The model under review builds one solid part; all positions refer to its coordinate system, in mm. A direction names the side the tool comes from. Round coordinates to 2 decimals unless told otherwise and drop trailing zeros. Use CSV: the item, a comma, the result in double quotes. Start each with the question number.
```python
from build123d import *

# Parameters (mm, degrees)
SKETCH3_R           = 0.95
SKETCH3_W           = 4.2
SKETCH3_H           = 8
SKETCH3_H_2         = 6
BOSS_EXTRUDE3_DEPTH = 2


with BuildPart() as part:
    # Sketch3 → Boss-Extrude3 (new body)
    with BuildSketch(Plane.XY):
        with BuildLine():
            Line((0, 94.006448831), (0, 86.061448831))
            ThreePointArc((0, 86.061448831), (0.585786438, 84.647235269), (2, 84.061448831))
            Line((2, 84.061448831), (4, 84.061448831))
            Line((4, 84.061448831), (4, 78.061448831))
            Line((4, 78.061448831), (2, 78.061448831))
            ThreePointArc((2, 78.061448831), (0.585786438, 77.475662393), (0, 76.061448831))
            Line((0, 76.061448831), (0, 60.606448831))
            ThreePointArc((0, 60.606448831), (0.585786438, 59.192235269), (2, 58.606448831))
            Line((2, 58.606448831), (4, 58.606448831))
            Line((4, 58.606448831), (4, 50.606448831))
            Line((4, 50.606448831), (2, 50.606448831))
            ThreePointArc((2, 50.606448831), (0.585786438, 50.020662393), (0, 48.606448831))
            Line((0, 48.606448831), (0, 26.346448831))
            ThreePointArc((0, 26.346448831), (0.585786438, 24.932235269), (2, 24.346448831))
            Line((2, 24.346448831), (4, 24.346448831))
            Line((4, 24.346448831), (4, 12.346448831))
            Line((4, 12.346448831), (6, 12.346448831))
            Line((6, 12.346448831), (6, 24.346448831))
            Line((6, 24.346448831), (10.2, 24.346448831))
            Line((10.2, 24.346448831), (10.2, 12.346448831))
            Line((10.2, 12.346448831), (12.2, 12.346448831))
            Line((12.2, 12.346448831), (12.2, 24.346448831))
            Line((12.2, 24.346448831), (14.2, 24.346448831))
            ThreePointArc((14.2, 24.346448831), (15.614213562, 24.932235269), (16.2, 26.346448831))
            Line((16.2, 26.346448831), (16.2, 48.606448831))
            ThreePointArc((16.2, 48.606448831), (15.614213562, 50.020662393), (14.2, 50.606448831))
            Line((14.2, 50.606448831), (12.2, 50.606448831))
            Line((12.2, 50.606448831), (12.2, 58.606448831))
            Line((12.2, 58.606448831), (14.2, 58.606448831))
            ThreePointArc((14.2, 58.606448831), (15.614213562, 59.192235269), (16.2, 60.606448831))
            Line((16.2, 60.606448831), (16.2, 76.061448831))
            ThreePointArc((16.2, 76.061448831), (15.614213562, 77.475662393), (14.2, 78.061448831))
            Line((14.2, 78.061448831), (12.2, 78.061448831))
            Line((12.2, 78.061448831), (12.2, 84.061448831))
            Line((12.2, 84.061448831), (14.2, 84.061448831))
            ThreePointArc((14.2, 84.061448831), (15.614213562, 84.647235269), (16.2, 86.061448831))
            Line((16.2, 86.061448831), (16.2, 94.006448831))
            Line((16.2, 94.006448831), (0, 94.006448831))
        make_face()
        with Locations((6, 33.846448831)):
            Circle(SKETCH3_R, mode=Mode.SUBTRACT)
        with Locations((10.2, 33.846448831)):
            Circle(SKETCH3_R, mode=Mode.SUBTRACT)
        with Locations((2.75, 86.061448831)):
            Circle(SKETCH3_R, mode=Mode.SUBTRACT)
        with Locations((10.2, 41.166448831)):
            Circle(SKETCH3_R, mode=Mode.SUBTRACT)
        with Locations((13.45, 48.106448831)):
            Circle(SKETCH3_R, mode=Mode.SUBTRACT)
        with Locations((2.75, 92.061448831)):
            Circle(SKETCH3_R, mode=Mode.SUBTRACT)
        with Locations((13.45, 86.061448831)):
            Circle(SKETCH3_R, mode=Mode.SUBTRACT)
        with Locations((2.75, 61.106448831)):
            Circle(SKETCH3_R, mode=Mode.SUBTRACT)
        with Locations((13.45, 61.106448831)):
            Circle(SKETCH3_R, mode=Mode.SUBTRACT)
        with Locations((2.75, 75.561448831)):
            Circle(SKETCH3_R, mode=Mode.SUBTRACT)
        with Locations((13.45, 26.846448831)):
            Circle(SKETCH3_R, mode=Mode.SUBTRACT)
        with Locations((13.45, 75.561448831)):
            Circle(SKETCH3_R, mode=Mode.SUBTRACT)
        with Locations((13.45, 92.061448831)):
            Circle(SKETCH3_R, mode=Mode.SUBTRACT)
        with Locations((2.75, 26.846448831)):
            Circle(SKETCH3_R, mode=Mode.SUBTRACT)
        with Locations((6, 41.106448831)):
            Circle(SKETCH3_R, mode=Mode.SUBTRACT)
        with Locations((2.75, 48.106448831)):
            Circle(SKETCH3_R, mode=Mode.SUBTRACT)
        with Locations((8.1, 54.606448831)):
            Rectangle(SKETCH3_W, SKETCH3_H, mode=Mode.SUBTRACT)
        with Locations((8.1, 81.061448831)):
            Rectangle(SKETCH3_W, SKETCH3_H_2, mode=Mode.SUBTRACT)
    extrude(amount=BOSS_EXTRUDE3_DEPTH)


solid = part.part
```
1. The part is to be moulded in two halves that separate along X. For faces 5 (the face through (2.63, 62.05, 0.99)), 6 (the face through (0, 90, 1)), 7 (the face through (8, 94.006, 1)), 8 (the face through (15.63, 77.46, 0.99)), say which applies: pulls with the +X half, pulls with the -X half, needs draft (parallel to the pull), parting line crosses it, or undercut.
2. For line 1 along Y through (x, z) = (7, 1.1); line 2 along X through (y, z) = (20.5, 1.75); line 3 along X through (y, z) = (60.5, 1.1), list the stretches that pass through material, from the lowest coordinate up. Write a range as from..to.
3. For faces 1 (the face through (8, 78.061, 1)), 2 (the face through (4, 18, 1)), 3 (the face through (12.2, 81, 1)), 4 (the face through (3, 84.061, 1)), list the 3-axis set-ups (+Z, -Z, +X, -X, +Y, -Y) from which the entire face can be reached by the end or side of a thin tool; tool diameter is ignored.
4. Clearance check with flat-ended pins moving along their axes: P1, Ø1, axis at x = 13.5, z = 1.5, coming from the -Y side; P2, Ø1.5, axis at x = 6, y = 33.85, coming from the -Z side. State where each tip first meets the part, or that it passes through.
5. Take a section at A-A, the plane x = 13.45. Count the separate pieces of the cut face and the enclosed holes in it, then the cut area to 3 significant figures.
Results:
1,face 5,"undercut"
1,face 6,"pulls with the -X half"
1,face 7,"needs draft"
1,face 8,"pulls with the +X half"
2,line 1,"24.35..50.61, 58.61..78.06, 84.06..94.01"
2,line 2,"4..6, 10.2..12.2"
2,line 3,"0..2.02, 3.48..12.72, 14.18..16.2"
3,face 1,"+Z, -Z"
3,face 2,"+Z, -Z, -X, -Y"
3,face 3,"+Z, -Z, +X"
3,face 4,"+Z, -Z, -X"
4,P1,"y = 24.35"
4,P2,"through"
5,separate pieces,"9"
5,enclosed holes,"0"
5,area,"88.5 mm²"
